Work out the finished part from the listing and answer in its coordinate system (mm). Face numbers are marked on the shaded views. A direction names the side the tool comes from. Give positions to 0.01 mm unless a question says otherwise; leave off trailing zeros. Order: outer loops, then holes, each group sorted by start corner. A loop starts at its lowest first (then second) coordinate and runs counter-clockwise, first axis right, second up. Notation, with made-up numbers: M -35.75,65.25 L -29.75,65.25 A20 ccw -29.75,77.25 Z; hole C 35,56.25 d5. An arc over 180 degrees is marked long. One line per item, written item: value.
from build123d import *

# Parameters (mm, degrees)
BOSS_EXTRUDE1_DEPTH = 17.25
BOSS_EXTRUDE2_DEPTH = 3
BOSS_EXTRUDE3_START = -20.25
BOSS_EXTRUDE3_DEPTH = 40.5
BOSS_EXTRUDE5_DEPTH = 3
BOSS_EXTRUDE6_DEPTH = 5
SKETCH9_W           = 1.8
SKETCH9_H           = 1
CUT_EXTRUDE2_DEPTH  = 20.25
BOSS_EXTRUDE7_DEPTH = 3


with BuildPart() as part:
    # Sketch1 → Boss-Extrude1 (new body)
    # profile 1 of 3: a face of its own
    with BuildSketch(Plane(origin=(0, 0, 0), x_dir=(0, 0, -1), z_dir=(1, 0, 0))):
        Polygon((0, 0), (5, 0), (5, -1.7), (7, -1.7), (7, 0), (38, 0), (57, 18.348086721), (57, -4), (33.8, -4), (33.8, -7.6), (30.2, -7.6), (30.2, -4), (0, -4), align=None)
        Polygon((54.5, 14.543701193), (39.43955654, 0), (54.5, 0), align=None, mode=Mode.SUBTRACT)
    # profile 2 of 3: a face of its own
    with BuildSketch(Plane(origin=(0, 0, 0), x_dir=(0, 0, -1), z_dir=(1, 0, 0))):
        Polygon((26.795, -4), (26.795, -10.332233047), (25.027233047, -12.1), (25.027233047, -4), align=None)
    # profile 3 of 3: a face of its own
    with BuildSketch(Plane(origin=(0, 0, 0), x_dir=(0, 0, -1), z_dir=(1, 0, 0))):
        Polygon((37.205, -4), (37.205, -10.332233047), (38.972766953, -12.1), (38.972766953, -4), align=None)
    boss_extrude1 = extrude(amount=BOSS_EXTRUDE1_DEPTH)

    # Sketch3 → Boss-Extrude2 (add)
    with BuildSketch(Plane(origin=(17.25, 0, 0), x_dir=(0, 0, -1), z_dir=(1, 0, 0))):
        Polygon((57, -4), (57, 49), (49, 49), (7, 7), (7, -1.7), (5, -1.7), (5, 0), (0, 0), (0, -4), (25.027233047, -4), (25.027233047, -12.1), (26.795, -10.332233047), (26.795, -4), (30.2, -4), (30.2, -7.6), (33.8, -7.6), (33.8, -4), (37.205, -4), (37.205, -10.332233047), (38.972766953, -12.1), (38.972766953, -4), align=None)
        Polygon((9.5, 5.964466094), (9.5, 0), (34.401108651, 0), (54.5, 19.409273762), (54.5, 46.5), (50.035533906, 46.5), align=None, mode=Mode.SUBTRACT)
        Polygon((39.43955654, 0), (54.5, 0), (54.5, 14.543701193), align=None, mode=Mode.SUBTRACT)
    boss_extrude2 = extrude(amount=BOSS_EXTRUDE2_DEPTH)

    # Mirror1: Boss-Extrude1, Boss-Extrude2 across plane
    add(boss_extrude1.mirror(Plane(origin=(0, 0, 0), x_dir=(0, 0, 1), z_dir=(1, 0, 0))))
    add(boss_extrude2.mirror(Plane(origin=(0, 0, 0), x_dir=(0, 0, 1), z_dir=(1, 0, 0))))

    # Sketch1<3> → Boss-Extrude3 (add)
    with BuildSketch(Plane(origin=(0, 0, 0), x_dir=(0, 0, -1), z_dir=(1, 0, 0)).offset(BOSS_EXTRUDE3_START)):
        Polygon((38, 0), (7, 0.270532902), (7, 0), align=None)
        Polygon((5, 0.287986637), (0, 0.331620976), (0, 0), (5, 0), align=None)
    extrude(amount=BOSS_EXTRUDE3_DEPTH)

    # Sketch6 → Boss-Extrude5 (add)
    with BuildSketch(Plane.ZY.offset(20.25)):
        Polygon((-37.205, 2.707686402), (-37.205, 33.669466094), (-38.972766953, 35.437233047), (-38.972766953, 4.414799105), align=None)
        Polygon((-26.795, 0.097784554), (-25.027233047, 0.113211622), (-25.027233047, 21.491699141), (-26.795, 23.259466094), align=None)
    boss_extrude5 = extrude(amount=-BOSS_EXTRUDE5_DEPTH)

    # Sketch8 → Boss-Extrude6 (add)
    # profile 1 of 2: a face of its own
    with BuildSketch(Plane.ZY.offset(20.25)):
        Polygon((-37.205, 33.669466094), (-37.205, 37.205), (-49, 49), (-57, 49), (-57, -4), (-38.972766953, -4), (-38.972766953, -12.1), (-37.205, -10.332233047), (-37.205, -4), (-37.205, 2.707686402), align=None)
        Polygon((-39.43955654, 0), (-54.5, 0), (-54.5, 14.543701193), align=None, mode=Mode.SUBTRACT)
        Polygon((-54.5, 19.409273762), (-54.5, 46.5), (-50.035533906, 46.5), (-38.972766953, 35.437233047), (-38.972766953, 4.414799105), align=None, mode=Mode.SUBTRACT)
    # profile 2 of 2: a face of its own
    with BuildSketch(Plane.ZY.offset(20.25)):
        Polygon((-5, 0.287986637), (-5, -1.7), (-7, -1.7), (-7, 7), (-26.795, 26.795), (-26.795, 23.259466094), (-26.795, 0.097784554), (-26.795, -4), (-26.795, -10.332233047), (-25.027233047, -12.1), (-25.027233047, -4), (0, -4), (0, 0.331620976), align=None)
        Polygon((-25.027233047, 0.113211622), (-25.027233047, 21.491699141), (-9.5, 5.964466094), (-9.5, 0.248715732), align=None, mode=Mode.SUBTRACT)
    boss_extrude6 = extrude(amount=BOSS_EXTRUDE6_DEPTH)

    # Sketch9 → Cut-Extrude2 (cut)
    with BuildSketch(Plane.ZY.offset(20.25)):
        Polygon((-28.445, 17.406308089), (-28.445, 24.909466094), (-30.215, 26.679466094), (-30.215, 21.679466094), (-37.205, 28.669466094), (-37.205, 26.166308089), align=None)
        Polygon((-26.795, 23.259466094), (-26.795, 26.795), (-28.445, 28.445), (-28.445, 24.909466094), align=None)
        with Locations((-27.695, -0.402215446)):
            Rectangle(SKETCH9_W, SKETCH9_H)
    cut_extrude2 = extrude(amount=-CUT_EXTRUDE2_DEPTH, mode=Mode.SUBTRACT)

    # Sketch9<3> → Boss-Extrude7 (add)
    with BuildSketch(Plane.ZY.offset(20.25)):
        Polygon((-28.445, 17.406308089), (-28.445, 24.909466094), (-30.215, 26.679466094), (-30.215, 21.679466094), (-37.205, 28.669466094), (-37.205, 26.166308089), align=None)
    boss_extrude7 = extrude(amount=-BOSS_EXTRUDE7_DEPTH)

    # Mirror2: Boss-Extrude5, Boss-Extrude6, Cut-Extrude2, Boss-Extrude7 across plane
    add(boss_extrude5.mirror(Plane(origin=(0, 0, 0), x_dir=(0, 0, 1), z_dir=(1, 0, 0))))
    add(boss_extrude6.mirror(Plane(origin=(0, 0, 0), x_dir=(0, 0, 1), z_dir=(1, 0, 0))))
    add(cut_extrude2.mirror(Plane(origin=(0, 0, 0), x_dir=(0, 0, 1), z_dir=(1, 0, 0))), mode=Mode.SUBTRACT)
    add(boss_extrude7.mirror(Plane(origin=(0, 0, 0), x_dir=(0, 0, 1), z_dir=(1, 0, 0))))


solid = part.part
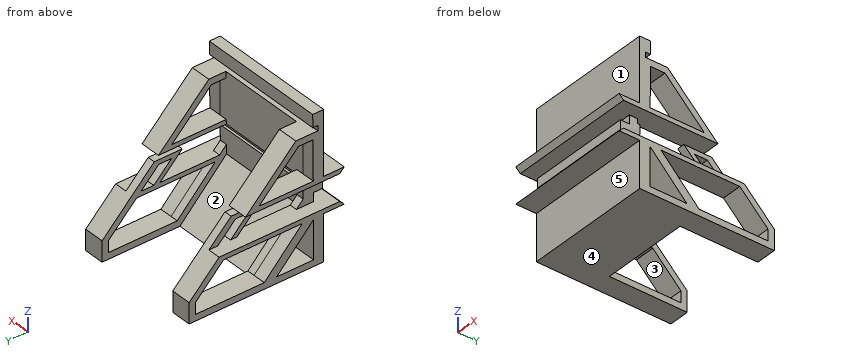
(1) Given P1, Ø1, axis at x = 14, y = 3, coming from the +Z side; P2, Ø14.5, axis at x = 2, z = -47, coming from the -Y side; P3, Ø1.8, axis at x = 0.5, y = -6, coming from the +Z side, each flat-ended and moving along its own axis, determine where each tip first touches the part or whether it passes through.
Findings:
P1: stops at z = -40.59
P2: stops at y = -4
P3: stops at z = -25.03
(2) Which of the six approach directions +Z, -Z, +X, -X, +Y, -Y give full straight-line access (tool end or side, diameter ignored) to the marked faces 3, 4 and 5?
Findings:
face 3: +X, -X
face 4: -Z, +X, -X, +Y, -Y
face 5: -Z, +X, -X, -Y
(3) Determine the mould class of the marked faces 1 and 2 for opening direction X: pulls with the +X half, pulls with the -X half, needs draft (parallel to the pull), parting line crosses it, or undercut.
Findings:
face 1: needs draft
face 2: undercut
(4) Section C-C, the plane x = 15 is taken. Give the vertices of the cut face in (y, z) (3 decimals), then the cut area to 3 significant figures.
Findings:
outline: M -12.1,-38.973 L -4,-38.973 L -4,-57 L 18.348,-57 L 0,-38 L 0.082,-28.595 L -0.902,-28.595 L -0.902,-26.795 L 0.098,-26.795 L 0.271,-7 L -1.7,-7 L -1.7,-5 L 0.288,-5 L 0.332,0 L -4,0 L -4,-25.027 L -12.1,-25.027 L -10.332,-26.795 L -4,-26.795 L -4,-30.2 L -7.6,-30.2 L -7.6,-33.8 L -4,-33.8 L -4,-37.205 L -10.332,-37.205 Z; hole M 0,-54.5 L 14.544,-54.5 L 0,-39.44 Z
area: 332 mm^2
(5) Section D-D, the plane y = 15.5 is taken. Give the number of separate pieces and of enclosed holes in the cut face, then the cut area to 3 significant figures.
Findings:
separate pieces: 7
enclosed holes: 0
area: 320 mm^2
(6) Find the intervals of material crossed by probe 1 along X at (y, z) = (0.5, -26.5); probe 2 along Z at (x, y) = (-20.5, 28) (3 decimals); probe 3 along Z at (x, y) = (-18.5, 22) (3 decimals), in increasing order. Write a range as from..to.
Findings:
probe 1: x = -25.25..-17.25, 17.25..25.25
probe 2: z = -57..-54.5, -38.973..-37.205
probe 3: z = -57..-54.5, -38.973..-37.205, -33.039..-30.536, -30.215..-28.445, -26.795..-22
(7) Section A-A, the plane y = 38.5 is taken. Give the vertices of the cut face in (x, z).
Findings:
outline: M -25.25,-57 L -17.25,-57 L -17.25,-54.5 L -25.25,-54.5 Z; M -25.25,-42.04 L -17.25,-42.04 L -17.25,-38.5 L -25.25,-38.5 Z; M 17.25,-57 L 25.25,-57 L 25.25,-54.5 L 17.25,-54.5 Z; M 17.25,-42.04 L 25.25,-42.04 L 25.25,-38.5 L 17.25,-38.5 Z
(8) Section B-B, the plane z = -14.5 is taken. Give the vertices of the cut face in (x, y).
Findings:
outline: M -25.25,-4 L 25.25,-4 L 25.25,0.21 L -25.25,0.21 Z; M -25.25,10.96 L -17.25,10.96 L -17.25,14.5 L -25.25,14.5 Z; M 17.25,10.96 L 25.25,10.96 L 25.25,14.5 L 17.25,14.5 Z
